Input: part model. Units: mm. Frame: model coordinates. A direction names the side the tool comes from. Coordinates: 2 decimals unless noted, no trailing zeros. Write each loop counter-clockwise with the first axis right and the second up, starting at its lowest first coordinate (ties: lowest second). Pieces come first, ordered by that corner, then holes.
1) Set-up query: faces 4 (the flat face through (28, 1, 10)), 5 (the flat face through (-35, 1, 0)), 6 (the flat face through (-28, 1, 10)). Return all of +Z, -Z, +X, -X, +Y, -Y with unobstructed straight access to the full face (end or side cutting, diameter ignored); none if empty.
2) Pin query (flat end, axial travel): pin 1 Ø1.5 at (y, z) = (0.5, 15) entering from +X (3 decimals); pin 2 Ø1 at (y, z) = (1.5, 42.5) entering from +X; pin 3 Ø0.9 at (x, y) = (28, 2) entering from +Z. Return the tip coordinate at first contact, or that it passes through.
3) Line query: L1, parallel to X at y = 1.15, z = 0; L2, parallel to X at y = 2.45, z = 55. Output: solid intervals per line, ascending.
4) Section query A-A (x = 0). Output: boundary loops of the cut face in (y, z), then the cut area to 3 significant figures.
5) Section query C-C (y = 1.9). Output: boundary loops of the cut face in (x, z).
6) Section query B-B (z = 25). Output: boundary loops of the cut face in (x, y), then the cut area to 3 significant figures.
7) Section query D-D (z = 0). Output: boundary loops of the cut face in (x, y).
8) Draft query along Z for faces 1 (the flat face through (-16, 1, 23)), 2 (the cylindrical face through (26.77, 1.48, 1.13)), 3 (the flat face through (35, 1, 0)). Return one class per face: pulls with the +Z half, pulls with the -Z half, needs draft (parallel to the pull), parting line crosses it, or undercut.
from build123d import *

# Parameters (mm, degrees)
SKETCH_1_R      = 2.1
EXTRUDE_1_DEPTH = 3
FILLET_1_R      = 3


with BuildPart() as part:
    # 草图1 → 凸台-拉伸1 (new body)
    # profile 1 of 3: a face of its own
    with BuildSketch(Plane(origin=(0, 0, 0), x_dir=(1, 0, 0), z_dir=(0, 1, 0))):
        Polygon((10, -10), (35, -10), (35, 10), (-35, 10), (-35, -10), (-10, -10), (-10, -60), (10, -60), align=None)
        with Locations(Location((0, -50, 0), (0, 0, 270))):
            Circle(SKETCH_1_R, mode=Mode.SUBTRACT)
        with Locations(Location((0, -25, 0), (0, 0, 270))):
            Circle(SKETCH_1_R, mode=Mode.SUBTRACT)
        with Locations(Location((-25, 0, 0), (0, 0, 270))):
            Circle(SKETCH_1_R, mode=Mode.SUBTRACT)
        with Locations(Location((25, 0, 0), (0, 0, 270))):
            Circle(SKETCH_1_R, mode=Mode.SUBTRACT)
        with Locations(Location((0, 0, 0), (0, 0, 270))):
            Circle(SKETCH_1_R, mode=Mode.SUBTRACT)
    # profile 2 of 3: a face of its own
    with BuildSketch(Plane(origin=(0, 0, 0), x_dir=(1, 0, 0), z_dir=(0, 1, 0))):
        Polygon((-10, -10), (-22.5, -10), (-10, -35), align=None)
    # profile 3 of 3: a face of its own
    with BuildSketch(Plane(origin=(0, 0, 0), x_dir=(1, 0, 0), z_dir=(0, 1, 0))):
        Polygon((10, -35), (22.5, -10), (10, -10), align=None)
    extrude(amount=EXTRUDE_1_DEPTH)

    # 圆角1
    fillet_1_edges = [part.edges().sort_by_distance(p)[0] for p in [
        (10, 1.5, 35),
        (10, 1.5, 60),
        (-10, 1.5, 60),
        (-10, 1.5, 35),
        (-22.5, 1.5, 10),
        (-35, 1.5, 10),
        (-35, 1.5, -10),
        (35, 1.5, -10),
        (35, 1.5, 10),
        (22.5, 1.5, 10),
    ]]
    fillet(fillet_1_edges, radius=FILLET_1_R)


solid = part.part
Answer:
1. face 4: +Z, +X, +Y, -Y
1. face 5: +Z, -Z, -X, +Y, -Y
1. face 6: +Z, -X, +Y, -Y
2. pin 1: stops at x = 20.375
2. pin 2: stops at x = 10
2. pin 3: stops at z = 10
3. L1: x = -35 to -27.1, -22.9 to -2.1, 2.1 to 22.9, 27.1 to 35
3. L2: x = -10 to 10
4. outline: (0, -10) - (3, -10) - (3, -2.1) - (0, -2.1) - close; (0, 2.1) - (3, 2.1) - (3, 22.9) - (0, 22.9) - close; (0, 27.1) - (3, 27.1) - (3, 47.9) - (0, 47.9) - close; (0, 52.1) - (3, 52.1) - (3, 60) - (0, 60) - close
4. area: 172 mm2
5. outline: (-35, -7) arc R3 ccw to (-32, -10) - (32, -10) arc R3 ccw to (35, -7) - (35, 7) arc R3 ccw to (32, 10) - (24.35, 10) arc R3 cw to (21.67, 11.66) - (10.32, 34.37) arc R3 cw to (10, 35.71) - (10, 57) arc R3 ccw to (7, 60) - (-7, 60) arc R3 ccw to (-10, 57) - (-10, 35.71) arc R3 cw to (-10.32, 34.37) - (-21.67, 11.66) arc R3 cw to (-24.35, 10) - (-32, 10) arc R3 ccw to (-35, 7) - close; hole circle Ø4.2 at (-25, 0); hole circle Ø4.2 at (0, 0); hole circle Ø4.2 at (0, 25); hole circle Ø4.2 at (0, 50); hole circle Ø4.2 at (25, 0)
6. outline: (-15, 0) - (-2.1, 0) - (-2.1, 3) - (-15, 3) - close; (2.1, 0) - (15, 0) - (15, 3) - (2.1, 3) - close
6. area: 77.4 mm2
7. outline: (-35, 0) - (-27.1, 0) - (-27.1, 3) - (-35, 3) - close; (-22.9, 0) - (-2.1, 0) - (-2.1, 3) - (-22.9, 3) - close; (2.1, 0) - (22.9, 0) - (22.9, 3) - (2.1, 3) - close; (27.1, 0) - (35, 0) - (35, 3) - (27.1, 3) - close
8. face 1: pulls with the +Z half
8. face 2: undercut
8. face 3: needs draft
